Could you check a few things on this model? Use its own coordinates, in mm. Face numbers are marked on the shaded views. A direction names the side the tool comes from. Coordinates: 2 decimals unless noted, no trailing zeros. Order: outer loops, then holes, each group sorted by start corner. A loop starts at its lowest first (then second) coordinate and runs counter-clockwise, first axis right, second up. Notation, with made-up numbers: M -2,19 L 50,19 A23 cw 50,47 Z; hole C 8,65 d7. An arc over 180 degrees is marked long. Write item = value, one per line. Start each with the question number.
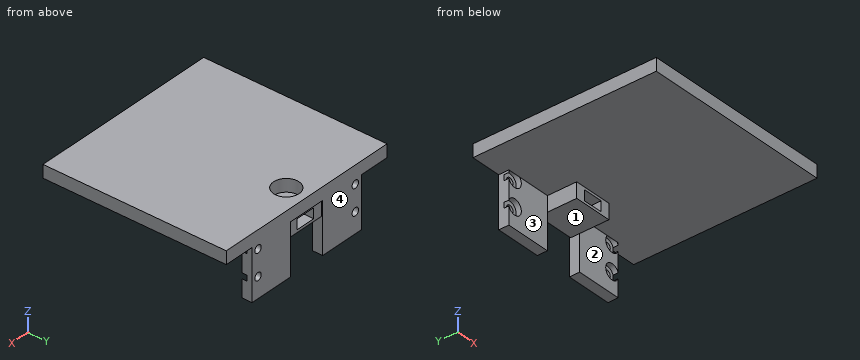
from build123d import *

# Parameters (mm, degrees)
SKETCH074_W     = 75
SKETCH074_H     = 72
SKETCH074_R     = 5
PAD027_DEPTH    = 5
SKETCH076_W     = 15
SKETCH076_H     = 15
PAD029_DEPTH    = 6
SKETCH077_W     = 7.8
SKETCH077_H     = 4
POCKET047_DEPTH = 15
SKETCH086_W     = 18
SKETCH086_H     = 4
PAD033_DEPTH    = 20
SKETCH087_R     = 1.5
POCKET053_DEPTH = 5
SKETCH088_R     = 3
POCKET054_DEPTH = 2


with BuildPart() as part:
    # Sketch074 → Pad027 (new body)
    with BuildSketch(Plane.XY):
        with Locations((0, -1)):
            Rectangle(SKETCH074_W, SKETCH074_H)
        with Locations((0, 27)):
            Circle(SKETCH074_R, mode=Mode.SUBTRACT)
    extrude(amount=PAD027_DEPTH)

    # Sketch076 → Pad029 (join)
    with BuildSketch(Plane(origin=(0, 0, 0), x_dir=(1, 0, 0), z_dir=(0, 0, -1))):
        with Locations((0, -27)):
            Rectangle(SKETCH076_W, SKETCH076_H)
    extrude(amount=PAD029_DEPTH)

    # Sketch077 (on Face8 of Pad029) → Pocket047 (cut)
    with BuildSketch(Plane(origin=(0, 34.5, 0), x_dir=(-1, 0, 0), z_dir=(0, 1, 0))):
        with Locations((0, -3)):
            Rectangle(SKETCH077_W, SKETCH077_H)
    extrude(amount=-POCKET047_DEPTH, mode=Mode.SUBTRACT)

    # Sketch086 (on Face4 of Pocket047) → Pad033 (join)
    with BuildSketch(Plane(origin=(0, 0, 0), x_dir=(1, 0, 0), z_dir=(0, 0, -1))):
        with Locations((-16.5, -33)):
            Rectangle(SKETCH086_W, SKETCH086_H)
        with Locations((16.5, -33)):
            Rectangle(SKETCH086_W, SKETCH086_H)
    extrude(amount=PAD033_DEPTH)

    # Sketch087 (on Face15 of Pad033) → Pocket053 (cut)
    with BuildSketch(Plane.XZ.offset(-31)):
        with Locations((-22.7, -2)):
            Circle(SKETCH087_R)
        with Locations((-22.7, -12)):
            Circle(SKETCH087_R)
    pocket053 = extrude(amount=-POCKET053_DEPTH, mode=Mode.SUBTRACT)

    # Sketch088 (on Face15 of Pocket053) → Pocket054 (cut)
    with BuildSketch(Plane.XZ.offset(-31)):
        with Locations((-22.7, -2)):
            Circle(SKETCH088_R)
        with Locations((-22.7, -12)):
            Circle(SKETCH088_R)
    pocket054 = extrude(amount=-POCKET054_DEPTH, mode=Mode.SUBTRACT)

    # Mirrored004: Pocket053, Pocket054 across Sketch087 V_Axis
    add(pocket053.mirror(Plane(origin=(0, 31, 0), x_dir=(0, -1, 0), z_dir=(1, 0, 0))), mode=Mode.SUBTRACT)
    add(pocket054.mirror(Plane(origin=(0, 31, 0), x_dir=(0, -1, 0), z_dir=(1, 0, 0))), mode=Mode.SUBTRACT)


with BuildPart() as part_1:
    # Body010 placement: moved
    add(part.part.moved(Location((0, 0, 30))))


solid = part_1.part
(1) Please list where these lines run through material, in increasing order: probe 1 along Z at (x, y) = (-22.7, 32.05); probe 2 along X at (y, z) = (32.4, 18); probe 3 along X at (y, z) = (20, 24.5). Write a range as from..to.
(2) Imagine slicing it at B-B on y = 27. List the corners of the cut face in (x, z) for me.
(3) For the marked faces 1, 2, 3 and 4, which set-ups out of +Z, -Z, +X, -X, +Y, -Y let a thin tool reach every point of the face, with its end or its side?
(4) Imagine slicing it at A-A on z = 18. List the corners of the cut face in (x, y) for me, plus the area to 3 significant figures.
(5) Imagine slicing it at C-C on x = 0. List the corners of the cut face in (y, z) for me, plus the area to 3 significant figures.
(6) Imagine slicing it at D-D on x = -22.7. List the corners of the cut face in (y, z) for me, plus the area to 3 significant figures.
(7) Will these pins go through, and if not, where does the flat tip stop? P1, Ø1.5, axis at x = -9, y = -11.5, coming from the -Z side; P2, Ø2, axis at y = 33, z = 15, coming from the +X side; P3, Ø2, axis at x = 4.5, z = 21.5, coming from the +Y side; P4, Ø7, axis at x = -22.7, z = 18, coming from the -Y side.
Response:
q1.probe_1 = 10..15, 21..25, 31..35
q1.probe_2 = -19.7..-7.5, 7.5..19.7
q1.probe_3 = -7.5..7.5
q2.outline = M -37.5,30 L -7.5,30 L -7.5,24 L 7.5,24 L 7.5,30 L 37.5,30 L 37.5,35 L 5,35 L 5,30 L -5,30 L -5,35 L -37.5,35 Z; hole M -3.9,25 L 3.9,25 L 3.9,29 L -3.9,29 Z
q3.face_1 = -Z, +Y, -Y
q3.face_2 = -Z, +X, -Y
q3.face_3 = -Z, -X, -Y
q3.face_4 = +Z, -Z, +X, -X, +Y
q4.outline = M -25.5,33 L -24.2,33 L -24.2,35 L -25.5,35 Z; M -21.2,33 L -19.7,33 L -19.7,31 L -7.5,31 L -7.5,35 L -21.2,35 Z; M 7.5,31 L 19.7,31 L 19.7,33 L 21.2,33 L 21.2,35 L 7.5,35 Z; M 24.2,33 L 25.5,33 L 25.5,35 L 24.2,35 Z
q4.area = 109 mm2
q5.outline = M -37,30 L 19.5,30 L 19.5,29 L 34.5,29 L 34.5,30 L 35,30 L 35,35 L 32,35 L 32,30 L 22,30 L 22,35 L -37,35 Z; M 19.5,24 L 34.5,24 L 34.5,25 L 19.5,25 Z
q5.area = 340 mm2
q6.outline = M -37,30 L 31,30 L 31,31 L 33,31 L 33,29.5 L 35,29.5 L 35,35 L -37,35 Z; M 31,10 L 35,10 L 35,16.5 L 33,16.5 L 33,15 L 31,15 Z; M 31,21 L 33,21 L 33,19.5 L 35,19.5 L 35,26.5 L 33,26.5 L 33,25 L 31,25 Z
q6.area = 404 mm2
q7.P1 = 30
q7.P2 = 25.5
q7.P3 = through
q7.P4 = 31
